Work out the finished part from the listing and answer in its coordinate system (mm). Face numbers are marked on the shaded views. Coordinates: 2 decimals unless noted, no trailing zeros. Loops run counter-clockwise (first coordinate to the right, second up) from the corner with the lowest first, then second, coordinate; pieces in that order, holes last.
```python
from build123d import *

# Parameters (mm, degrees)
PARED_B_CHUMACERA_J5_START          = -10.525
CROQUIS1_W                          = 52
CROQUIS1_H                          = 60.6
PARED_B_CHUMACERA_J5_DEPTH          = 6.35
PARED_B_CHUMACERA_J5_REDONDEO_START = -10.525
CROQUIS2_R                          = 26
PARED_B_CHUMACERA_J5_REDONDEO_DEPTH = 6.35
PASO_PERNO_Y_ROSCA_M4_KFL08_START   = -10.525
CROQUIS3_R                          = 4.5
CROQUIS3_R_2                        = 1.65
PASO_PERNO_Y_ROSCA_M4_KFL08_DEPTH   = 6.35
ROSCA_M3_ESCUADRAS_START            = -10.525
CROQUIS4_R                          = 1.25
ROSCA_M3_ESCUADRAS_DEPTH            = 6.35
PASADORES_D4_START                  = 275.95
CROQUIS5_R                          = 2
PASADORES_D4_DEPTH                  = 8
ROSCA_M3_BASES_CINCHO_START         = -10.525
CROQUIS6_R                          = 1.25
ROSCA_M3_BASES_CINCHO_DEPTH         = 6.35


with BuildPart() as part:
    # Croquis1 → Pared_B_chumacera_J5 (new body)
    with BuildSketch(Plane(origin=(0, 0, 0), x_dir=(1, 0, 0), z_dir=(0, 1, 0)).offset(PARED_B_CHUMACERA_J5_START)):
        with Locations((152.4, -306.25)):
            Rectangle(CROQUIS1_W, CROQUIS1_H)
    extrude(amount=PARED_B_CHUMACERA_J5_DEPTH)

    # Croquis2 → Pared_B_chumacera_J5_redondeo (add)
    with BuildSketch(Plane(origin=(0, 0, 0), x_dir=(1, 0, 0), z_dir=(0, 1, 0)).offset(PARED_B_CHUMACERA_J5_REDONDEO_START)):
        with Locations((152.4, -336.55)):
            Circle(CROQUIS2_R)
    extrude(amount=PARED_B_CHUMACERA_J5_REDONDEO_DEPTH)

    # Croquis3 → Paso_perno_y_rosca_M4_KFL08 (cut)
    with BuildSketch(Plane(origin=(0, 0, 0), x_dir=(1, 0, 0), z_dir=(0, 1, 0)).offset(PASO_PERNO_Y_ROSCA_M4_KFL08_START)):
        with Locations(Location((152.4, -336.55, 0), (0, 0, 90))):
            Circle(CROQUIS3_R)
        with Locations(Location((152.4, -355.05, 0), (0, 0, 90))):
            Circle(CROQUIS3_R_2)
        with Locations(Location((152.4, -318.05, 0), (0, 0, 90))):
            Circle(CROQUIS3_R_2)
    extrude(amount=PASO_PERNO_Y_ROSCA_M4_KFL08_DEPTH, mode=Mode.SUBTRACT)

    # Croquis4 → Rosca_M3_escuadras (cut)
    with BuildSketch(Plane(origin=(0, 0, 0), x_dir=(1, 0, 0), z_dir=(0, 1, 0)).offset(ROSCA_M3_ESCUADRAS_START)):
        with Locations(Location((134.4, -290.95, 0), (0, 0, 90))):
            Circle(CROQUIS4_R)
        with Locations(Location((170.4, -290.95, 0), (0, 0, 90))):
            Circle(CROQUIS4_R)
    extrude(amount=ROSCA_M3_ESCUADRAS_DEPTH, mode=Mode.SUBTRACT)

    # Croquis5 → Pasadores_D4 (cut)
    with BuildSketch(Plane.XY.offset(PASADORES_D4_START)):
        with Locations((130.4, -7.35)):
            Circle(CROQUIS5_R)
        with Locations((174.4, -7.35)):
            Circle(CROQUIS5_R)
    extrude(amount=PASADORES_D4_DEPTH, mode=Mode.SUBTRACT)

    # Croquis6 → Rosca_M3_bases_cincho (cut)
    with BuildSketch(Plane(origin=(0, 0, 0), x_dir=(1, 0, 0), z_dir=(0, 1, 0)).offset(ROSCA_M3_BASES_CINCHO_START)):
        with Locations(Location((152.4, -296, 0), (0, 0, 90))):
            Circle(CROQUIS6_R)
    extrude(amount=ROSCA_M3_BASES_CINCHO_DEPTH, mode=Mode.SUBTRACT)


solid = part.part
```
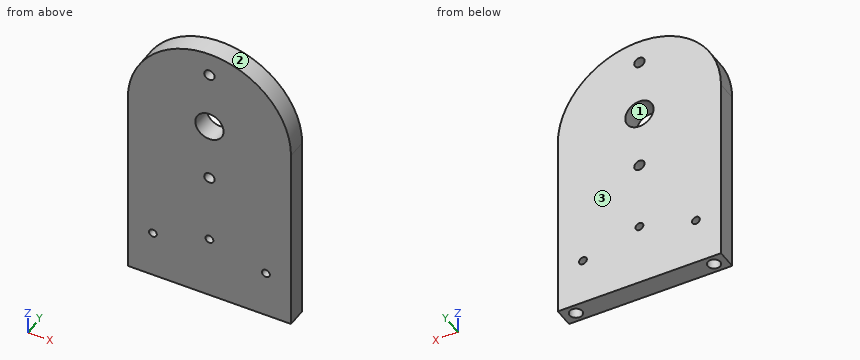
1. A cutting plane is placed at C-C, the plane z = 283. Give the vertices of the cut face in (x, y) (3 decimals).
2. Each of these flat-tipped pins is pushed along its axis until it touches: P1, Ø3, axis at x = 152.4, z = 355.05, coming from the -Y side (1 decimal); P2, Ø3, axis at x = 174.4, y = -7.35, coming from the -Z side. Where does it stop, or does it pass through?
3. A cutting plane is placed at D-D, the plane x = 134.4. Give the vertices of the cut face in (y, z) (3 decimals), then the cut area to 3 significant figures.
4. A cutting plane is placed at B-B, the plane x = 152.4. Give the vertices of the cut face in (y, z) (3 decimals), then the cut area to 3 significant figures.
5. Straight lines are drawn through the part: probe 1 along Z at (x, y) = (152.4, -8.75); probe 2 along X at (y, z) = (-8.25, 290.95); probe 3 along X at (y, z) = (-8, 296). For each, find the intervals that lie inside material, in ascending order.
6. Determine the mould class of the marked faces 1, 2 and 3 for opening direction X: released by +X, released by -X, zero draft, split by the parting line, or undercut.
7. A cutting plane is placed at A-A, the plane z = 318.05. Give the vertices of the cut face in (x, y) (3 decimals).
Answers below:
1. outline: (126.4, -10.525) - (178.4, -10.525) - (178.4, -4.175) - (126.4, -4.175) - close; hole circle Ø4 at (130.4, -7.35); hole circle Ø4 at (174.4, -7.35)
2. P1: passes through
2. P2: stops at z = 283.95
3. outline: (-10.525, 275.95) - (-4.175, 275.95) - (-4.175, 289.7) - (-10.525, 289.7) - close; (-10.525, 292.2) - (-4.175, 292.2) - (-4.175, 355.312) - (-10.525, 355.312) - close
3. area: 488 mm2
4. outline: (-10.525, 275.95) - (-4.175, 275.95) - (-4.175, 294.75) - (-10.525, 294.75) - close; (-10.525, 297.25) - (-4.175, 297.25) - (-4.175, 316.4) - (-10.525, 316.4) - close; (-10.525, 319.7) - (-4.175, 319.7) - (-4.175, 332.05) - (-10.525, 332.05) - close; (-10.525, 341.05) - (-4.175, 341.05) - (-4.175, 353.4) - (-10.525, 353.4) - close; (-10.525, 356.7) - (-4.175, 356.7) - (-4.175, 362.55) - (-10.525, 362.55) - close
4. area: 435 mm2
5. probe 1: z = 275.95 to 294.75, 297.25 to 316.4, 319.7 to 332.05, 341.05 to 353.4, 356.7 to 362.55
5. probe 2: x = 126.4 to 133.15, 135.65 to 169.15, 171.65 to 178.4
5. probe 3: x = 126.4 to 151.15, 153.65 to 178.4
6. face 1: undercut
6. face 2: split by the parting line
6. face 3: zero draft
7. outline: (126.4, -10.525) - (150.75, -10.525) - (150.75, -4.175) - (126.4, -4.175) - close; (154.05, -10.525) - (178.4, -10.525) - (178.4, -4.175) - (154.05, -4.175) - close
